from build123d import *

# Parameters (mm, degrees)
SKETCH2_W          = 10.7
SKETCH2_H          = 7.5
SKETCH2_H_2        = 12.5
SKETCH2_W_2        = 44.2
SKETCH2_H_3        = 5
SKETCH2_W_3        = 24
SKETCH2_H_4        = 6
CUT_EXTRUDE2_REACH = 108.104
SKETCH5_R          = 6.061151683
FILLET2_R          = 3.5
FILLET3_R          = 3.5


with BuildPart() as part:
    # Sketch2 → Revolve5 (revolve)
    with BuildSketch(Plane(origin=(0, 0, 0), x_dir=(1, 0, 0), z_dir=(0, 1, 0))):
        with Locations((29.205555556, -41.25)):
            Rectangle(SKETCH2_W, SKETCH2_H)
        Polygon((34.555555556, -15), (23.855555556, -15), (23.855555556, -20), (23.855555556, -25), (34.555555556, -25), align=None)
        Polygon((23.855555556, 25), (23.855555556, 20), (23.855555556, 15), (34.555555556, 15), (34.555555556, 25), align=None)
        with Locations((29.205555556, 41.25)):
            Rectangle(SKETCH2_W, SKETCH2_H)
        with Locations((29.205555556, -31.25)):
            Rectangle(SKETCH2_W, SKETCH2_H_2)
        with Locations((1.755555556, -17.5)):
            Rectangle(SKETCH2_W_2, SKETCH2_H_3)
        with Locations((1.755555556, 17.5)):
            Rectangle(SKETCH2_W_2, SKETCH2_H_3)
        Polygon((-20.344444444, -15), (-26.344444444, -15), (-26.344444444, -19), (-26.344444444, -25), (-20.344444444, -25), (-20.344444444, -20), align=None)
        Polygon((-20.344444444, 25), (-26.344444444, 25), (-26.344444444, 19), (-26.344444444, 15), (-20.344444444, 15), (-20.344444444, 20), align=None)
        with Locations((-38.344444444, 22)):
            Rectangle(SKETCH2_W_3, SKETCH2_H_4)
        with Locations((-38.344444444, -22)):
            Rectangle(SKETCH2_W_3, SKETCH2_H_4)
    revolve(axis=Axis((-47.361111111, 0, 0), (1, 0, 0)))

    # Sketch5 → Cut-Extrude2 (cut, up to next)
    with BuildSketch(Plane(origin=(34.555555556, 0, 0), x_dir=(0, 0, -1), z_dir=(1, 0, 0)), mode=Mode.PRIVATE) as cut_extrude2_sk1:
        with Locations((0, 30)):
            Circle(SKETCH5_R)
    cut_extrude2_tool1 = extrude(cut_extrude2_sk1.sketch, amount=-CUT_EXTRUDE2_REACH, mode=Mode.PRIVATE) & part.part
    # Sketch5 → Cut-Extrude2 (cut, up to next)
    with BuildSketch(Plane(origin=(34.555555556, 0, 0), x_dir=(0, 0, -1), z_dir=(1, 0, 0)), mode=Mode.PRIVATE) as cut_extrude2_sk2:
        with Locations((30, 0)):
            Circle(SKETCH5_R)
    cut_extrude2_tool2 = extrude(cut_extrude2_sk2.sketch, amount=-CUT_EXTRUDE2_REACH, mode=Mode.PRIVATE) & part.part
    # Sketch5 → Cut-Extrude2 (cut, up to next)
    with BuildSketch(Plane(origin=(34.555555556, 0, 0), x_dir=(0, 0, -1), z_dir=(1, 0, 0)), mode=Mode.PRIVATE) as cut_extrude2_sk3:
        with Locations((0, -30)):
            Circle(SKETCH5_R)
    cut_extrude2_tool3 = extrude(cut_extrude2_sk3.sketch, amount=-CUT_EXTRUDE2_REACH, mode=Mode.PRIVATE) & part.part
    # Sketch5 → Cut-Extrude2 (cut, up to next)
    with BuildSketch(Plane(origin=(34.555555556, 0, 0), x_dir=(0, 0, -1), z_dir=(1, 0, 0)), mode=Mode.PRIVATE) as cut_extrude2_sk4:
        with Locations((-30, 0)):
            Circle(SKETCH5_R)
    cut_extrude2_tool4 = extrude(cut_extrude2_sk4.sketch, amount=-CUT_EXTRUDE2_REACH, mode=Mode.PRIVATE) & part.part
    add(cut_extrude2_tool1.solids().sort_by_distance((34.555556, 30, 0))[0], mode=Mode.SUBTRACT)
    add(cut_extrude2_tool2.solids().sort_by_distance((34.555556, 0, -30))[0], mode=Mode.SUBTRACT)
    add(cut_extrude2_tool3.solids().sort_by_distance((34.555556, -30, 0))[0], mode=Mode.SUBTRACT)
    add(cut_extrude2_tool4.solids().sort_by_distance((34.555556, 0, 30))[0], mode=Mode.SUBTRACT)

    # Fillet2
    fillet2_edges = [part.edges().sort_by_distance(p)[0] for p in [
        (-20.344444444, 0, -25),
    ]]
    fillet(fillet2_edges, radius=FILLET2_R)

    # Fillet3
    # the kernel refuses this fillet: 3.5 mm, written as the material it adds along each edge
    with BuildSketch(Plane(origin=(23.855555556, 0, 0), x_dir=(0, 0, 1), z_dir=(0, 1, 0))) as fillet3_piece_1:
        with BuildLine():
            CenterArc((20 + FILLET3_R, -FILLET3_R), FILLET3_R, 90, 90)
            Line((20 + FILLET3_R, 0), (20, 0))
            Line((20, 0), (20, -FILLET3_R))
        make_face()
    revolve(axis=Axis((23.855555556, 0, 0), (1, 0, 0)))
    # the kernel refuses this fillet: 3.5 mm, written as the material it takes off along each edge
    with BuildSketch(Plane(origin=(-50.344444444, 0, 0), x_dir=(0, 0, -1), z_dir=(0, 1, 0))) as fillet3_2_piece_1:
        with BuildLine():
            CenterArc((25 - FILLET3_R, -FILLET3_R), FILLET3_R, 0, 90)
            Line((25 - FILLET3_R, 0), (25, 0))
            Line((25, 0), (25, -FILLET3_R))
        make_face()
    revolve(axis=Axis((-50.344444444, 0, 0), (-1, 0, 0)), mode=Mode.SUBTRACT)
    with BuildSketch(Plane(origin=(23.855555556, 0, 0), x_dir=(0, 0, 1), z_dir=(0, 1, 0))) as fillet3_2_piece_2:
        with BuildLine():
            CenterArc((45 - FILLET3_R, FILLET3_R), FILLET3_R, 270, 90)
            Line((45, FILLET3_R), (45, 0))
            Line((45, 0), (45 - FILLET3_R, 0))
        make_face()
    revolve(axis=Axis((23.855555556, 0, 0), (1, 0, 0)), mode=Mode.SUBTRACT)


solid = part.part
Verification items for the finished model (mm, model axes). A direction names the side the tool comes from. Give positions to 0.01 mm unless a question says otherwise; leave off trailing zeros. Write each loop counter-clockwise with the first axis right and the second up, starting at its lowest first coordinate (ties: lowest second). Pieces come first, ordered by that corner, then holes. Notation, with made-up numbers: (83.25, -40) -> (107.25, -40) arc R26 ccw to (107.25, -6) -> close; hole circle Ø11 at (-16, 77.25). An arc over 180 degrees is marked (long way). Use CSV: the item, a comma, the result in double quotes.
(1) Sectioned sample at C-C (x = -22.5). Record the cut outline in (y, z), plus the area to 3 significant figures.
Derived:
outline,"circle Ø49.46 at (0, 0); hole circle Ø30 at (0, 0)"
area,"1,210 mm^2"
(2) Release check for a two-part mould opening along Z. For faces 1 (the flat face through (-20.344, 13, 16)), 2 (the cylindrical face through (29.28, -2.32, -35.6)), 3 (the cylindrical face through (31.006, -39.923, -20.765)) record: +Z half, -Z half, draft (parallel to the pull), parting line (faces both ways), or undercut.
Derived:
face 1,"draft"
face 2,"undercut"
face 3,"parting line"
(3) Go/stop test with flat-tipped pins: pin 1 (6 mm diameter, centred on x = -35, z = -1, fed in from -Y); pin 2 (19 mm diameter, centred on y = -2.5, z = 3, fed in from -X); pin 3 (1.5 mm diameter, centred on x = -34.5, y = -1.5, fed in from +Z); pin 4 (16 mm diameter, centred on y = 0, z = -30, fed in from -X). Record where each tip stops, or that it passes through.
Derived:
pin 1,"stops at y = -25"
pin 2,"passes through"
pin 3,"stops at z = 24.99"
pin 4,"stops at x = -50.31"
(4) Sectioned sample at D-D (x = 25.5). Record the cut outline in (y, z).
Derived:
outline,"circle Ø88.94 at (0, 0); hole circle Ø12.12 at (-30, 0); hole circle Ø30 at (0, 0); hole circle Ø12.12 at (0, -30); hole circle Ø12.12 at (0, 30); hole circle Ø12.12 at (30, 0)"
(5) Material ranges on L1, parallel to Y at x = 28, z = 0; L2, parallel to Y at x = 29, z = 4; L3, parallel to X at y = 26, z = 9, recorded low to high.
Derived:
L1,"y = -45 to -36.06, -23.94 to -15, 15 to 23.94, 36.06 to 45"
L2,"y = -44.82 to -34.55, -25.45 to -14.46, 14.46 to 25.45, 34.55 to 44.82"
L3,"x = 23.86 to 34.56"
(6) Set-up check for faces 4 (the flat face through (34.556, 11, -11)), 5 (the cylindrical face through (-35.183, -7.509, 23.846)), 6 (the flat face through (-50.344, 16, 11)), 7 (the cylindrical face through (29.28, 1.82, 24.22)), 8 (the cylindrical face through (0.29, 19.524, -4.336)): record each of +Z, -Z, +X, -X, +Y, -Y from which the full face is reachable in a straight line by a thin tool's end or side.
Derived:
face 4,"+Z, -Z, +X, +Y, -Y"
face 5,"-X"
face 6,"+Z, -Z, -X, +Y, -Y"
face 7,"+X"
face 8,"none"
(7) Sectioned sample at A-A (y = 0). Give the number of separate pieces and of enclosed holes in the cut face, plus the area to 3 significant figures.
Derived:
separate pieces,"4"
enclosed holes,"0"
area,"1,220 mm^2"
